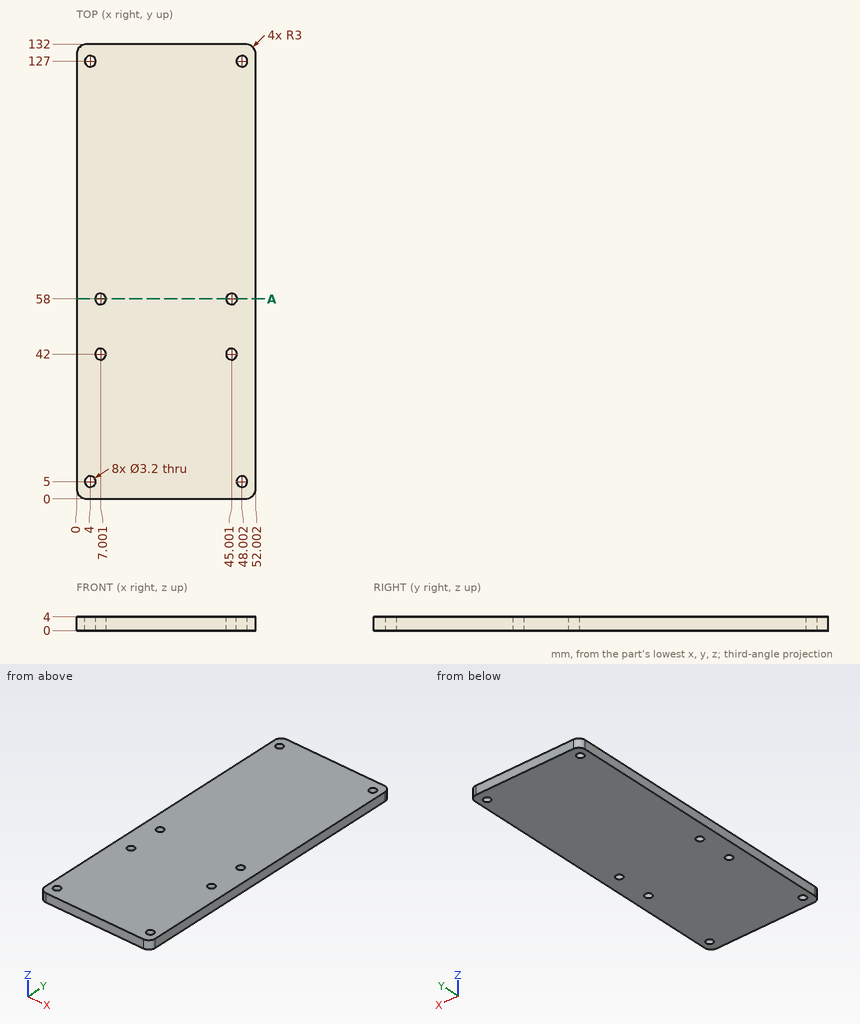
Design review of the part shown in the three views and the two pictorial views. Dimensions are in mm from the part's minimum x, y and z. Give positions to 0.01 mm unless a question says otherwise; leave off trailing zeros. Write each loop counter-clockwise with the first axis right and the second up, starting at its lowest first coordinate (ties: lowest second). Pieces come first, ordered by that corner, then holes. Notation, with made-up numbers: M 23.25,-26.75 L 66.25,-26.75 A21 ccw 66.25,-17.75 Z; hole C 13.5,-35 d5. An arc over 180 degrees is marked long. Return JSON: item names as keys, results as strings. Group by question number.
Item 1: Take a section at A-A (y = 58). Give the boundary of the cut face in (x, z).
Item 2: Wall thickness on line 1 along Y through (x, z) = (4, 0.55); line 2 along X through (y, z) = (127, 1.2); line 3 along X through (y, z) = (57.5, 0.35): over which ranges is each line inside the solid? List them lowest first.
Item 3: Clearance check with a flat-ended pin moving along its axis: pin 1 Ø4 at (x, y) = (48, 127) entering from -Z. State where the tip first meets the part, or that it passes through.
Return value:
{
 "1": {"outline": "M 0,0 L 5.4,0 L 5.4,4 L 0,4 Z; M 8.6,0 L 43.4,0 L 43.4,4 L 8.6,4 Z; M 46.6,0 L 52,0 L 52,4 L 46.6,4 Z"},
 "2": {"line 1": "y = 0 to 3.4, 6.6 to 125.4, 128.6 to 132", "line 2": "x = 0 to 2.4, 5.6 to 46.4, 49.6 to 52", "line 3": "x = 0 to 5.48, 8.52 to 43.48, 46.52 to 52"},
 "3": {"pin 1": "stops at z = 0"}
}
